Can you work these out from the model? Positions are in its coordinate system, mm. Face numbers are marked on the shaded views. Round coordinates to 2 decimals unless told otherwise and drop trailing zeros. Loops run counter-clockwise (first coordinate to the right, second up) from the corner with the lowest first, then second, coordinate; pieces in that order, holes last.
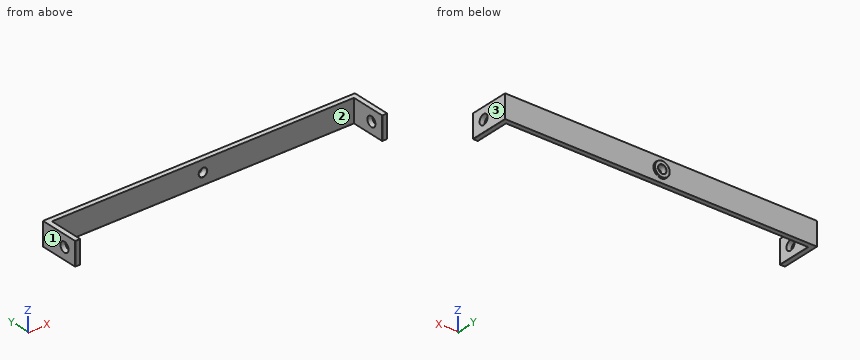
```python
from build123d import *

# Parameters (mm, degrees)
BOSS_EXTRUDE1_DEPTH     = 3.5
SKETCH2_R               = 1.25
CUT_EXTRUDE1_DEPTH      = 13
SKETCH3_R               = 2.25
SKETCH3_R_2             = 1.25
BOSS_EXTRUDE2_DEPTH     = 0.5
SKETCH4_R               = 1.5
CUT_EXTRUDE2_DEPTH      = 48
CUT_EXTRUDE2_DEPTH_BACK = 48
FILLET1_R               = 0.075


with BuildPart() as part:
    # Sketch1 → Boss-Extrude1 (new body, symmetric)
    with BuildSketch(Plane.XY):
        Polygon((-47, 0), (47, 0), (47, -12), (45.5, -12), (45.5, -1.5), (-45.5, -1.5), (-45.5, -12), (-47, -12), align=None)
    extrude(amount=BOSS_EXTRUDE1_DEPTH, both=True)

    # Sketch2 → Cut-Extrude1 (cut, through all)
    with BuildSketch(Plane(origin=(0, 0, 0), x_dir=(1, 0, 0), z_dir=(0, 1, 0))):
        Circle(SKETCH2_R)
    extrude(amount=-CUT_EXTRUDE1_DEPTH, mode=Mode.SUBTRACT)

    # Sketch3 → Boss-Extrude2 (add)
    with BuildSketch(Plane(origin=(0, 0, 0), x_dir=(1, 0, 0), z_dir=(0, 1, 0))):
        Circle(SKETCH3_R)
        Circle(SKETCH3_R_2, mode=Mode.SUBTRACT)
    extrude(amount=BOSS_EXTRUDE2_DEPTH)

    # Sketch4 → Cut-Extrude2 (cut, two sides)
    with BuildSketch(Plane(origin=(0, 0, 0), x_dir=(0, 0, -1), z_dir=(1, 0, 0))) as cut_extrude2_sk:
        with Locations((0, -8)):
            Circle(SKETCH4_R)
    extrude(amount=CUT_EXTRUDE2_DEPTH, mode=Mode.SUBTRACT)
    extrude(cut_extrude2_sk.sketch, amount=-CUT_EXTRUDE2_DEPTH_BACK, mode=Mode.SUBTRACT)

    # Fillet1
    fillet1_edges = [part.edges().sort_by_distance(p)[0] for p in [
        (-45.5, -6.75, -3.5),
        (0, -1.5, -3.5),
        (-2.25, 0, 0),
        (47, -12, 0),
        (47, 0, 0),
        (-47, -12, 0),
        (-45.5, -12, 0),
        (-45.5, -1.5, 0),
        (45.5, -1.5, 0),
        (45.5, -12, 0),
        (-46.25, -12, 3.5),
        (45.5, -6.75, -3.5),
        (-46.25, -12, -3.5),
        (47, -6, -3.5),
        (46.25, -12, -3.5),
        (-1.25, -1.5, 0),
        (-2.25, 0.5, 0),
        (-1.25, 0.5, 0),
    ]]
    fillet(fillet1_edges, radius=FILLET1_R)


solid = part.part
```
(1) If I drill on line 1 (X direction, y = -0.8, z = 0); line 2 (X direction, y = -10.25, z = 3); line 3 (Y direction, x = -46.15, z = 0), over which ranges is the centre line in solid material (lowest first)?
(2) Suppose I cut it at B-B (y = -8). Write out the boundary of the cut face in (x, z) (3 decimals), then the cut area to 3 significant figures.
(3) Suppose I cut it at C-C (x = 0). Write out the boundary of the cut face in (y, z) (3 decimals).
(4) Suppose I cut it at A-A (y = -2.5). Write out the boundary of the cut face in (x, z) (3 decimals), then the cut area to 3 significant figures.
(5) For pin 1 (4 mm diameter, centred on x = -33, z = -3, fed in from +Y); pin 2 (2 mm diameter, centred on x = 16.5, z = 0, fed in from -Y), each with a flat end and sliding along its axis, tell me the tip position at first contact or that it passes through.
(6) We'd pull the mould along X, two halves only. Please class the marked faces 1, 2 and 3: released by +X, released by -X, zero draft, split by the parting line, or undercut.
(7) Suppose I cut it at D-D (x = -26.5). Write out the boundary of the cut face in (y, z) (3 decimals).
Check result:
1. line 1: x = -47 to -1.25, 1.25 to 47
1. line 2: x = -47 to -45.5, 45.5 to 47
1. line 3: y = -12 to -9.5, -6.5 to 0
2. outline: (-47, -3.5) - (-45.575, -3.5) arc R0.075 ccw to (-45.5, -3.425) - (-45.5, -1.5) - (-47, -1.5) - close; (-47, 1.5) - (-45.5, 1.5) - (-45.5, 3.5) - (-47, 3.5) - close; (45.5, -3.425) arc R0.075 ccw to (45.575, -3.5) - (46.925, -3.5) arc R0.075 ccw to (47, -3.425) - (47, -1.5) - (45.5, -1.5) - close; (45.5, 1.5) - (47, 1.5) - (47, 3.5) - (45.5, 3.5) - close
2. area: 12.0 mm2
3. outline: (-1.5, -3.425) arc R0.075 ccw to (-1.425, -3.5) - (0, -3.5) - (0, -2.325) arc R0.075 cw to (0.075, -2.25) - (0.425, -2.25) arc R0.075 ccw to (0.5, -2.175) - (0.5, -1.325) arc R0.075 ccw to (0.425, -1.25) - (-1.425, -1.25) arc R0.075 ccw to (-1.5, -1.325) - close; (-1.5, 1.325) arc R0.075 ccw to (-1.425, 1.25) - (0.425, 1.25) arc R0.075 ccw to (0.5, 1.325) - (0.5, 2.175) arc R0.075 ccw to (0.425, 2.25) - (0.075, 2.25) arc R0.075 cw to (0, 2.325) - (0, 3.5) - (-1.5, 3.5) - close
4. outline: (-47, -3.5) - (-45.575, -3.5) arc R0.075 ccw to (-45.5, -3.425) - (-45.5, 3.5) - (-47, 3.5) - close; (45.5, -3.425) arc R0.075 ccw to (45.575, -3.5) - (46.925, -3.5) arc R0.075 ccw to (47, -3.425) - (47, 3.5) - (45.5, 3.5) - close
4. area: 21.0 mm2
5. pin 1: stops at y = 0
5. pin 2: stops at y = -1.5
6. face 1: released by -X
6. face 2: undercut
6. face 3: released by +X
7. outline: (-1.5, -3.425) arc R0.075 ccw to (-1.425, -3.5) - (0, -3.5) - (0, 3.5) - (-1.5, 3.5) - close
